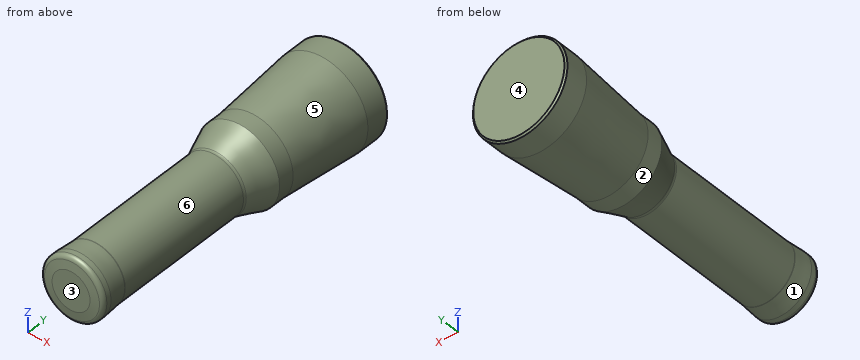
```python
from build123d import *

# Parameters (mm, degrees)
SFAZOWANIE1_SIZE = 1


with BuildPart() as part:
    # Szkic1 → Obrót5 (revolve)
    with BuildSketch(Plane.XY, mode=Mode.PRIVATE) as obr_t5_sk:
        with BuildLine():
            Line((-18.236763899, 104.399774637), (-18.236763899, 17.739774637))
            ThreePointArc((-18.236763899, 17.739774637), (-18.239809764, 17.565277154), (-18.248943647, 17.390992269))
            Line((-18.248943647, 17.390992269), (-19.02, 6.364372704))
            Line((-19.02, 6.364372704), (-19.02, 3.307537954))
            ThreePointArc((-19.02, 3.307537954), (-18.362673282, 1.561062759), (-16.716937778, 0.681398805))
            Line((-16.716937778, 0.681398805), (-11.5412, 0))
            Line((-11.5412, 0), (0, 0))
            Line((0, 0), (0, 198.039004786))
            Line((0, 198.039004786), (-28.72, 198.039004786))
            Line((-28.72, 198.039004786), (-28.72, 183.039004786))
            Line((-28.72, 183.039004786), (-24.7, 133.039004786))
            Line((-24.7, 133.039004786), (-24.7, 123.039004786))
            Line((-24.7, 123.039004786), (-18.538300795, 106.109875354))
            ThreePointArc((-18.538300795, 106.109875354), (-18.312725134, 105.268015526), (-18.236763899, 104.399774637))
        make_face()
    revolve(obr_t5_sk.sketch.rotate(Axis((0, 198.039004786, 0), (0, -1, 0)), 270), axis=Axis((0, 198.039004786, 0), (0, -1, 0)))

    # Sfazowanie1
    sfazowanie1_edges = [part.edges().sort_by_distance(p)[0] for p in [
        (0, 198.039004786, -28.72),
    ]]
    chamfer(sfazowanie1_edges, length=SFAZOWANIE1_SIZE)


solid = part.part
```
The listing builds one solid part. Answer for the finished solid, in the listing's coordinates (mm). Face numbers are marked on the shaded views. A direction names the side the tool comes from. Round coordinates to 2 decimals unless told otherwise and drop trailing zeros. Write each loop counter-clockwise with the first axis right and the second up, starting at its lowest first coordinate (ties: lowest second). Pieces come first, ordered by that corner, then holes. Notation, with made-up numbers: (-14.5, 12.25) -> (18.5, 12.25) arc R22 cw to (18.5, 32.25) -> close; hole circle Ø7 at (52.25, -10). An arc over 180 degrees is marked (long way). Answer as a JSON object with one key per item and string values. Group by question number.
Q1. Section A-A (z = 0) is taken. Write down the section's boundary in (x, y), plus the area to 3 significant figures.
Q2. Each of these flat-tipped pins is pushed along its axis until it touches: pin 1 Ø12 at (y, z) = (76.5, -14.5) entering from -X; pin 2 Ø8 at (y, z) = (44.5, 14) entering from +X; pin 3 Ø10 at (x, y) = (-10, 82) entering from -Z. Where does it stop, or does it pass through?
Q3. Section B-B (x = 0) is taken. Write down the section's boundary in (y, z), plus the area to 3 significant figures.
Q4. Section C-C (y = 135) is taken. Write down the section's boundary in (x, z), plus the area to 3 significant figures.
Q5. Which of the six approach directions +Z, -Z, +X, -X, +Y, -Y give full straight-line access (tool end or side, diameter ignored) to the marked faces 5 and 6?
Q6. Determine the mould class of the marked faces 1, 2, 3 and 4 for opening direction Y: pulls with the +Y half, pulls with the -Y half, needs draft (parallel to the pull), parting line crosses it, or undercut.
Q7. Straight lines are drawn through the part: line 1 along Z through (x, y) = (1, 123.5); line 2 along Z through (x, y) = (7.5, 185); line 3 along X through (y, z) = (103.5, 7.5). For each, find the intervals that lie inside material, in ascending order.
Check values:
{
 "1": {"outline": "(-28.72, 183.04) -> (-24.7, 133.04) -> (-24.7, 123.04) -> (-18.54, 106.11) arc R5 cw to (-18.24, 104.4) -> (-18.24, 17.74) arc R5 cw to (-18.25, 17.39) -> (-19.02, 6.36) -> (-19.02, 3.31) arc R2.65 ccw to (-16.72, 0.68) -> (-11.54, 0) -> (11.54, 0) -> (16.72, 0.68) arc R2.65 ccw to (19.02, 3.31) -> (19.02, 6.36) -> (18.25, 17.39) arc R5 cw to (18.24, 17.74) -> (18.24, 104.4) arc R5 cw to (18.54, 106.11) -> (24.7, 123.04) -> (24.7, 133.04) -> (28.72, 183.04) -> (28.72, 197.04) -> (27.72, 198.04) -> (-27.72, 198.04) -> (-28.72, 197.04) -> close", "area": "8,640 mm^2"},
 "2": {"pin 1": "x = -16.13", "pin 2": "x = 15.25", "pin 3": "z = -17.54"},
 "3": {"outline": "(0, -11.54) -> (0.68, -16.72) arc R2.65 ccw to (3.31, -19.02) -> (6.36, -19.02) -> (17.39, -18.25) arc R5 cw to (17.74, -18.24) -> (104.4, -18.24) arc R5 cw to (106.11, -18.54) -> (123.04, -24.7) -> (133.04, -24.7) -> (183.04, -28.72) -> (197.04, -28.72) -> (198.04, -27.72) -> (198.04, 27.72) -> (197.04, 28.72) -> (183.04, 28.72) -> (133.04, 24.7) -> (123.04, 24.7) -> (106.11, 18.54) arc R5 cw to (104.4, 18.24) -> (17.74, 18.24) arc R5 cw to (17.39, 18.25) -> (6.36, 19.02) -> (3.31, 19.02) arc R2.65 ccw to (0.68, 16.72) -> (0, 11.54) -> close", "area": "8,640 mm^2"},
 "4": {"outline": "circle Ø49.72 at (0, 0)", "area": "1,940 mm^2"},
 "5": {"face 5": "-Y", "face 6": "none"},
 "6": {"face 1": "undercut", "face 2": "needs draft", "face 3": "pulls with the -Y half", "face 4": "pulls with the +Y half"},
 "7": {"line 1": "-24.68 to 24.68", "line 2": "-27.72 to 27.72", "line 3": "-16.62 to 16.62"}
}
